```python
from build123d import *

# Parameters (mm, degrees)
CROQUIS1_W              = 36
CROQUIS1_H              = 22.25
CROQUIS1_R              = 1.5
CROQUIS1_R_2            = 3.05
CROQUIS1_R_3            = 1.875
SALIENTE_EXTRUIR1_DEPTH = 1.5
CROQUIS2_R              = 1.5
CROQUIS2_W              = 10
CROQUIS2_H              = 1.5
SALIENTE_EXTRUIR2_DEPTH = 1
CROQUIS3_R              = 1.500000001
CROQUIS3_R_2            = 1.5
SALIENTE_EXTRUIR6_DEPTH = 0.9


with BuildPart() as part:
    # Croquis1 → Saliente-Extruir1 (new body)
    with BuildSketch(Plane.XY):
        Rectangle(CROQUIS1_W, CROQUIS1_H)
        with Locations((13.8, 8.745)):
            Circle(CROQUIS1_R, mode=Mode.SUBTRACT)
        with Locations(Location((13.8, -8.745, 0), (0, 0, 180))):
            Circle(CROQUIS1_R, mode=Mode.SUBTRACT)
        with Locations(Location((6.8, 0, 0), (0, 0, 180))):
            Circle(CROQUIS1_R_2, mode=Mode.SUBTRACT)
        with Locations((-13.8, -8.745)):
            Circle(CROQUIS1_R, mode=Mode.SUBTRACT)
        with Locations(Location((-13.8, 8.745, 0), (0, 0, 180))):
            Circle(CROQUIS1_R, mode=Mode.SUBTRACT)
        with Locations(Location((-4.2, 0, 0), (0, 0, 180))):
            Circle(CROQUIS1_R_3, mode=Mode.SUBTRACT)
    extrude(amount=SALIENTE_EXTRUIR1_DEPTH)

    # Croquis2 → Saliente-Extruir2 (add)
    # profile 1 of 4: a face of its own
    with BuildSketch(Plane.XZ.offset(11.125)):
        with BuildLine():
            Line((-5.5, -8.5), (-5.5, 0))
            Line((-5.5, 0), (-15.5, 0))
            Line((-15.5, 0), (-15.5, -8.5))
            ThreePointArc((-15.5, -8.5), (-10.5, -13.5), (-5.5, -8.5))
        make_face()
        with Locations((-10.5, -8.5)):
            Circle(CROQUIS2_R, mode=Mode.SUBTRACT)
    # profile 2 of 4: a face of its own
    with BuildSketch(Plane.XZ.offset(11.125)):
        with Locations((-10.5, 0.75)):
            Rectangle(CROQUIS2_W, CROQUIS2_H)
    # profile 3 of 4: a face of its own
    with BuildSketch(Plane.XZ.offset(11.125)):
        with BuildLine():
            Line((15.5, 0), (5.5, 0))
            Line((5.5, 0), (5.5, -8.5))
            ThreePointArc((5.5, -8.5), (10.5, -13.5), (15.5, -8.5))
            Line((15.5, -8.5), (15.5, 0))
        make_face()
        with Locations((10.5, -8.5)):
            Circle(CROQUIS2_R, mode=Mode.SUBTRACT)
    # profile 4 of 4: a face of its own
    with BuildSketch(Plane.XZ.offset(11.125)):
        with Locations((10.5, 0.75)):
            Rectangle(CROQUIS2_W, CROQUIS2_H)
    extrude(amount=SALIENTE_EXTRUIR2_DEPTH)

    # Croquis3 → Saliente-Extruir6 (add)
    # profile 1 of 2: a face of its own
    with BuildSketch(Plane(origin=(0, 11.125, 0), x_dir=(1, 0, 0), z_dir=(0, 1, 0))):
        with BuildLine():
            ThreePointArc((-17.865049678, -1.5), (0, -17.3), (17.865049678, -1.5))
            Line((17.865049678, -1.5), (-17.865049678, -1.5))
        make_face()
        with Locations(Location((-7.071067812, -4.871067812, 0), (0, 0, 180))):
            Circle(CROQUIS3_R, mode=Mode.SUBTRACT)
        with Locations(Location((0, -7.8, 0), (0, 0, 180))):
            Circle(CROQUIS3_R_2, mode=Mode.SUBTRACT)
        with Locations(Location((7.071067812, -4.871067812, 0), (0, 0, 180))):
            Circle(CROQUIS3_R_2, mode=Mode.SUBTRACT)
    # profile 2 of 2: a face of its own
    with BuildSketch(Plane(origin=(0, 11.125, 0), x_dir=(1, 0, 0), z_dir=(0, 1, 0))):
        with BuildLine():
            ThreePointArc((17.865049678, -1.5), (17.941399597, -0.751268579), (17.986383739, 0))
            Line((17.986383739, 0), (-17.986383739, 0))
            ThreePointArc((-17.986383739, 0), (-17.941399597, -0.751268579), (-17.865049678, -1.5))
            Line((-17.865049678, -1.5), (17.865049678, -1.5))
        make_face()
    extrude(amount=-SALIENTE_EXTRUIR6_DEPTH)


solid = part.part
```
The listing builds one solid part. Answer for the finished solid, in the listing's coordinates (mm). A direction names the side the tool comes from. Coordinates: 2 decimals unless noted, no trailing zeros. Write each loop counter-clockwise with the first axis right and the second up, starting at its lowest first coordinate (ties: lowest second). Pieces come first, ordered by that corner, then holes. Notation, with made-up numbers: (25.25, 40) -> (69.25, 40) arc R25 cw to (69.25, 61) -> close; hole circle Ø1 at (-34, 32.5). An arc over 180 degrees is marked (long way). Write each question's results on one line, items separated by ' | '. Start each with the question number.
1) Flat-ended cylindrical pins translate along their axes: pin 1 Ø5 at (x, z) = (0, 2.5) entering from -Y (3 decimals); pin 2 Ø3 at (y, z) = (1.5, 2) entering from -X; pin 3 Ø1.8 at (x, z) = (-7.07, 4.87) entering from -Y; pin 4 Ø5 at (y, z) = (-9, -5) entering from +X. Find the tip coordinate at first contact, or state that the pin passes through.
2) For a pull along Y with two mould halves and no side action, classify faces 3 (the flat face through (-18, 0, 1)), 4 (the cylindrical face through (13.108, -7.414, 0.74)), 5 (the flat face through (-17, -11.125, 1)) as +Y half, -Y half, draft (parallel to the pull), parting line (faces both ways), or undercut.
3) Straight lines are drawn through the part: probe 1 along Y at (x, z) = (13.8, 1.1) (3 decimals); probe 2 along Y at (x, z) = (11, -10) (3 decimals); probe 3 along Z at (x, y) = (-2.5, 7.25). For each, find the intervals that lie inside material, in ascending order.
4) A tool of negligible diameter and unlimited length cuts with its end or side. For faces 1 (the flat face through (-10.6, -11.125, -6.7)), 2 (the flat face through (18, 0, 1)), from which of +Z, -Z, +X, -X, +Y, -Y can it reach the whole face along a straight path? Write none if from no direction.
5) A cutting plane is placed at C-C (y = -9.75). Determine the outline of the cut face in (x, z).
6) A cutting plane is placed at A-A (x = 0). Determine the outline of the cut face in (y, z) (3 decimals), then the cut area to 3 significant figures.
7) A cutting plane is placed at B-B (z = -5). Determine the outline of the cut face in (x, y) (3 decimals).
8) A cutting plane is placed at D-D (y = -2.5). Determine the outline of the cut face in (x, z), then the cut area to 3 significant figures.
Values follow:
1) pin 1: y = -11.125 | pin 2: x = -18 | pin 3: through | pin 4: x = 15.5
2) face 3: draft | face 4: undercut | face 5: -Y half
3) probe 1: -12.125 to -10.245, -7.245 to 7.245, 10.225 to 11.125 | probe 2: -12.125 to -11.125 | probe 3: 0 to 1.5
4) face 1: -Z, +X, -X, +Y | face 2: +Z, -Z, +X, +Y, -Y
5) outline: (-18, 0) -> (-14.91, 0) -> (-14.91, 1.5) -> (-18, 1.5) -> close; (-12.69, 0) -> (12.69, 0) -> (12.69, 1.5) -> (-12.69, 1.5) -> close; (14.91, 0) -> (18, 0) -> (18, 1.5) -> (14.91, 1.5) -> close
6) outline: (-11.125, 0) -> (11.125, 0) -> (11.125, 6.3) -> (10.225, 6.3) -> (10.225, 1.5) -> (-11.125, 1.5) -> close; (10.225, 9.3) -> (11.125, 9.3) -> (11.125, 17.3) -> (10.225, 17.3) -> close | area: 44.9 mm²
7) outline: (-15.5, -12.125) -> (-5.5, -12.125) -> (-5.5, -11.125) -> (-15.5, -11.125) -> close; (5.5, -12.125) -> (15.5, -12.125) -> (15.5, -11.125) -> (5.5, -11.125) -> close
8) outline: (-18, 0) -> (5.05, 0) -> (5.05, 1.5) -> (-18, 1.5) -> close; (8.55, 0) -> (18, 0) -> (18, 1.5) -> (8.55, 1.5) -> close | area: 48.8 mm²
